from build123d import *

# Parameters (mm, degrees)
BOSS_EXTRUDE1_DEPTH = 3.175
FILLET1_R           = 5.08
SKETCH2_R           = 2.413
CUT_EXTRUDE1_DEPTH  = 3.175
SKETCH3_R           = 2.413
CUT_EXTRUDE2_DEPTH  = 3.175


with BuildPart() as part:
    # Sketch1 → Boss-Extrude1 (new body)
    with BuildSketch(Plane(origin=(0, 0, 0), x_dir=(1, 0, 0), z_dir=(0, 1, 0))):
        Polygon((0, 0), (393.7, 0), (196.85, 340.95420147), align=None)
    extrude(amount=BOSS_EXTRUDE1_DEPTH)

    # Fillet1
    fillet1_edges = [part.edges().sort_by_distance(p)[0] for p in [
        (196.85, 1.5875, -340.95420147),
        (393.7, 1.5875, 0),
        (0, 1.5875, 0),
    ]]
    fillet(fillet1_edges, radius=FILLET1_R)

    # Sketch2 → Cut-Extrude1 (cut)
    with BuildSketch(Plane(origin=(0, 3.175, 0), x_dir=(1, 0, 0), z_dir=(0, 1, 0))):
        with Locations((37.394976935, 21.59)):
            Circle(SKETCH2_R)
        with Locations((59.392022192, 34.29)):
            Circle(SKETCH2_R)
        with Locations((70.39054482, 40.64)):
            Circle(SKETCH2_R)
        with Locations((114.384635332, 66.04)):
            Circle(SKETCH2_R)
        with Locations((103.386112704, 59.69)):
            Circle(SKETCH2_R)
        with Locations((196.85, 297.77420147)):
            Circle(SKETCH2_R)
        with Locations((196.85, 272.37420147)):
            Circle(SKETCH2_R)
        with Locations((196.85, 259.67420147)):
            Circle(SKETCH2_R)
        with Locations((196.85, 221.57420147)):
            Circle(SKETCH2_R)
        with Locations((196.85, 208.87420147)):
            Circle(SKETCH2_R)
        with Locations((279.315364668, 66.04)):
            Circle(SKETCH2_R)
        with Locations((290.313887296, 59.69)):
            Circle(SKETCH2_R)
        with Locations((323.30945518, 40.64)):
            Circle(SKETCH2_R)
        with Locations((334.307977808, 34.29)):
            Circle(SKETCH2_R)
        with Locations((356.305023065, 21.59)):
            Circle(SKETCH2_R)
    extrude(amount=-CUT_EXTRUDE1_DEPTH, mode=Mode.SUBTRACT)

    # Sketch3 → Cut-Extrude2 (cut)
    with BuildSketch(Plane(origin=(0, 3.175, 0), x_dir=(1, 0, 0), z_dir=(0, 1, 0))):
        with BuildLine():
            Line((389.300590949, 7.62), (212.725, 313.4578949))
            Line((212.725, 313.4578949), (212.725, 0))
            Line((212.725, 0), (384.901181898, 0))
            ThreePointArc((384.901181898, 0), (389.300590949, 2.54), (389.300590949, 7.62))
        make_face()
        with Locations((290.313887296, 59.69)):
            Circle(SKETCH3_R, mode=Mode.SUBTRACT)
        with Locations((279.315364668, 66.04)):
            Circle(SKETCH3_R, mode=Mode.SUBTRACT)
        with Locations((323.30945518, 40.64)):
            Circle(SKETCH3_R, mode=Mode.SUBTRACT)
        with Locations((334.307977808, 34.29)):
            Circle(SKETCH3_R, mode=Mode.SUBTRACT)
        with Locations((356.305023065, 21.59)):
            Circle(SKETCH3_R, mode=Mode.SUBTRACT)
    extrude(amount=-CUT_EXTRUDE2_DEPTH, mode=Mode.SUBTRACT)


solid = part.part
The listing builds one solid part. Answer for the finished solid, in the listing's coordinates (mm). Give positions to 0.01 mm unless a question says otherwise; leave off trailing zeros. Order: outer loops, then holes, each group sorted by start corner. A loop starts at its lowest first (then second) coordinate and runs counter-clockwise, first axis right, second up. Notation, with made-up numbers: (78, -23.5) - (126, -23.5) arc R19 cw to (126, -5.5) - close; hole circle Ø3 at (52, 74.25). An arc over 180 degrees is marked (long way). Answer as CSV lines item,"result".
Q1. A cutting plane is placed at B-B, the plane z = -178. Determine the outline of the cut face in (x, y) (3 decimals), and give its area (3 significant figures).
Answer key:
outline,"(102.768, 0) - (212.725, 0) - (212.725, 3.175) - (102.768, 3.175) - close"
area,"349 mm^2"
Q2. Straight lines are drawn through the part: L1, parallel to Z at x = 196.85, y = 2.1; L2, parallel to X at y = 1.05, z = -34.29 (3 decimals); L3, parallel to Z at x = 57.5, y = 1.2. For each, find the intervals that lie inside material, in ascending order.
Answer key:
L1,"z = -335.87 to -300.19, -295.36 to -274.79, -269.96 to -262.09, -257.26 to -223.99, -219.16 to -211.29, -206.46 to 0"
L2,"x = 19.797 to 56.979, 61.805 to 212.725"
L3,"z = -99.59 to -35.79, -32.79 to 0"
Q3. A cutting plane is placed at A-A, the plane y = 1.5. Count the separate pieces of the cut face and the enclosed holes in it, and give its area (3 significant figures).
Answer key:
separate pieces,"1"
enclosed holes,"10"
area,"38,500 mm^2"
Q4. This flat-tipped pin is pushed along its axis until it touches: pin 1 Ø3 at (x, z) = (196.85, -221.57) entering from -Y. Where does it stop, or does it pass through?
Answer key:
pin 1,"passes through"
